Here's the drawing with two shaded views (mm, measured from the low corner). I have some questions. Round coordinates to 2 decimals unless told otherwise and drop trailing zeros. Loops run counter-clockwise (first coordinate to the right, second up) from the corner with the lowest first, then second, coordinate; pieces in that order, holes last. Notation, with made-up numbers: (-8.5, -31.75) - (37.5, -31.75) arc R23 cw to (37.5, 7.25) - close; hole circle Ø1 at (65.5, 81.25). An arc over 180 degrees is marked (long way). Use one line per item in the form item = value.
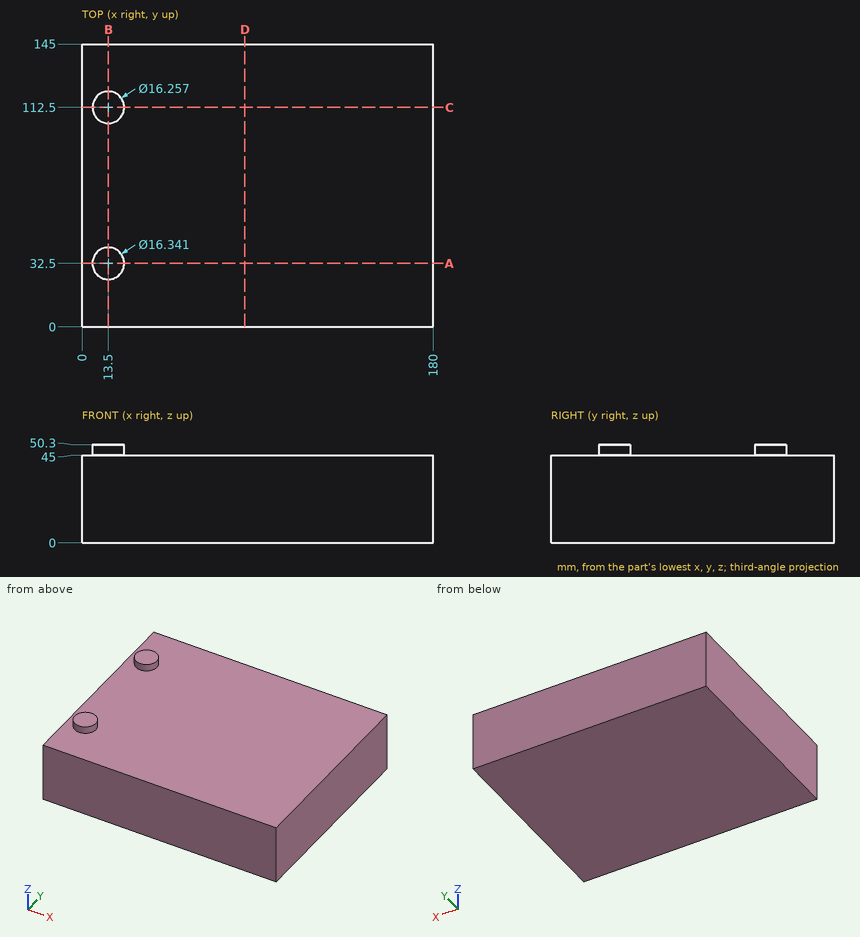
1. If we section it at C-C, the plane y = 112.5: Write out the boundary of the cut face in (x, z), plus the area to 3 significant figures.
Solution:
outline = (0, 0) - (180, 0) - (180, 45) - (21.63, 45) - (21.63, 50.3) - (5.37, 50.3) - (5.37, 45) - (0, 45) - close
area = 8,190 mm^2
2. If we section it at B-B, the plane x = 13.5: Write out the boundary of the cut face in (y, z), plus the area to 3 significant figures.
Solution:
outline = (0, 0) - (145, 0) - (145, 45) - (120.63, 45) - (120.63, 50.3) - (104.37, 50.3) - (104.37, 45) - (40.67, 45) - (40.67, 50.3) - (24.33, 50.3) - (24.33, 45) - (0, 45) - close
area = 6,700 mm^2
3. For P1, Ø10, axis at x = 46, y = 76.5, coming from the +Z side, with a flat end and sliding along its axis, tell me the tip position at first contact or that it passes through.
Solution:
P1 = 45
4. If we section it at D-D, the plane x = 83.5: Write out the boundary of the cut face in (y, z).
Solution:
outline = (0, 0) - (145, 0) - (145, 45) - (0, 45) - close
5. Please list where this line runs through material, in increasing order: line 1 along Z through (x, y) = (98, 9.5).
Solution:
line_1 = 0 to 45
6. If we section it at A-A, the plane y = 32.5: Write out the boundary of the cut face in (x, z), plus the area to 3 significant figures.
Solution:
outline = (0, 0) - (180, 0) - (180, 45) - (21.67, 45) - (21.67, 50.3) - (5.33, 50.3) - (5.33, 45) - (0, 45) - close
area = 8,190 mm^2
